Geometry check sheet. Reference: the model listing, model coordinates, mm. Face numbers are marked on the shaded views. A direction names the side the tool comes from. Round coordinates to 2 decimals unless told otherwise and drop trailing zeros. Write each loop counter-clockwise with the first axis right and the second up, starting at its lowest first coordinate (ties: lowest second). Pieces come first, ordered by that corner, then holes. Notation, with made-up numbers: (29, 38.25) -> (72, 38.25) arc R25 ccw to (72, 76.25) -> close; hole circle Ø4 at (49, 4). An arc over 180 degrees is marked (long way). Return JSON: item names as keys, results as strings. Group by question number.
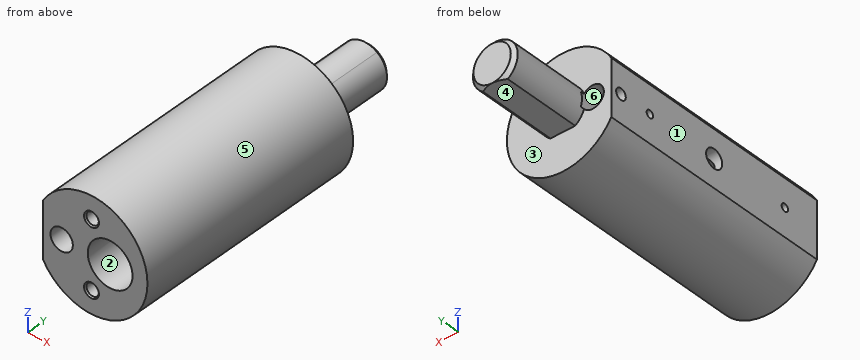
from build123d import *

# Parameters (mm, degrees)
BOSS_EXTRUDE1_DEPTH         = 22
BOSS_EXTRUDE2_DEPTH         = 64
SKETCH3_R                   = 3
CUT_EXTRUDE1_DEPTH          = 65
SKETCH4_R                   = 6
CUT_EXTRUDE2_DEPTH          = 52
M4_TAPPED_HOLE2_D           = 3.3
M4_TAPPED_HOLE2_DEPTH       = 16.8
M4_TAPPED_HOLE2_CSINK_D     = 4
M4_TAPPED_HOLE2_CSINK_ANGLE = 90
M4_TAPPED_HOLE2_TIP         = 0.991420021
SKETCH20_R                  = 2.5
SKETCH20_R_2                = 1.5
CUT_EXTRUDE3_DEPTH          = 5
SKETCH21_R                  = 1
CUT_EXTRUDE4_DEPTH          = 15
BOSS_EXTRUDE4_START         = -22
BOSS_EXTRUDE4_DEPTH         = 22
CUT_EXTRUDE5_DEPTH          = 22
CHAMFER1_SIZE               = 1


with BuildPart() as part:
    # Sketch1 → Boss-Extrude1 (new body)
    with BuildSketch(Plane(origin=(0, 0, 0), x_dir=(1, 0, 0), z_dir=(0, 1, 0))):
        with BuildLine():
            Line((-3.31662479, -5), (3.31662479, -5))
            ThreePointArc((3.31662479, -5), (0, 6), (-3.31662479, -5))
        make_face()
    extrude(amount=BOSS_EXTRUDE1_DEPTH)

    # Sketch2 → Boss-Extrude2 (add)
    with BuildSketch(Plane.XZ):
        with BuildLine():
            Line((-13, 7.483314774), (-13, -7.483314774))
            ThreePointArc((-13, -7.483314774), (15, 0), (-13, 7.483314774))
        make_face()
    extrude(amount=BOSS_EXTRUDE2_DEPTH)

    # Sketch3 → Cut-Extrude1 (cut)
    with BuildSketch(Plane.XZ.offset(64)):
        with Locations(Location((-8, 0, 0), (0, 0, 270))):
            Circle(SKETCH3_R)
    extrude(amount=-CUT_EXTRUDE1_DEPTH, mode=Mode.SUBTRACT)

    # Sketch4 → Cut-Extrude2 (cut)
    with BuildSketch(Plane(origin=(0, -64, 0), x_dir=(-1, 0, 0), z_dir=(0, -1, 0))):
        with Locations(Location((-5, 0, 0), (0, 0, 90))):
            Circle(SKETCH4_R)
    extrude(amount=-CUT_EXTRUDE2_DEPTH, mode=Mode.SUBTRACT)

    # M4 Tapped Hole2
    with Locations(Plane(origin=(0, -64, 0), x_dir=(-1, 0, 0), z_dir=(0, -1, 0))):
        with Locations((0, -9), (0, 9)):
            CounterSinkHole(M4_TAPPED_HOLE2_D / 2, M4_TAPPED_HOLE2_CSINK_D / 2, depth=M4_TAPPED_HOLE2_DEPTH, counter_sink_angle=M4_TAPPED_HOLE2_CSINK_ANGLE)
            with Locations((0, 0, -(M4_TAPPED_HOLE2_DEPTH + M4_TAPPED_HOLE2_TIP / 2))):  # 118° drill point
                Cone(0, M4_TAPPED_HOLE2_D / 2, M4_TAPPED_HOLE2_TIP, mode=Mode.SUBTRACT)

    # Sketch20 → Cut-Extrude3 (cut)
    with BuildSketch(Plane.ZY.offset(13)):
        with Locations((0, -32)):
            Circle(SKETCH20_R)
        with Locations((0, -3)):
            Circle(SKETCH20_R_2)
    extrude(amount=-CUT_EXTRUDE3_DEPTH, mode=Mode.SUBTRACT)

    # Sketch21 → Cut-Extrude4 (cut)
    with BuildSketch(Plane.ZY.offset(13)):
        with Locations((0, -12)):
            Circle(SKETCH21_R)
        with Locations((0, -54)):
            Circle(SKETCH21_R)
    extrude(amount=-CUT_EXTRUDE4_DEPTH, mode=Mode.SUBTRACT)

    # Sketch22 → Boss-Extrude4 (add)
    with BuildSketch(Plane(origin=(0, 22, 0), x_dir=(1, 0, 0), z_dir=(0, 1, 0)).offset(BOSS_EXTRUDE4_START)):
        with BuildLine():
            Line((3.31662479, -5), (-3.31662479, -5))
            ThreePointArc((-3.31662479, -5), (0, -6), (3.31662479, -5))
        make_face()
    extrude(amount=BOSS_EXTRUDE4_DEPTH)

    # Sketch23 → Cut-Extrude5 (cut)
    with BuildSketch(Plane(origin=(0, 22, 0), x_dir=(1, 0, 0), z_dir=(0, 1, 0))):
        Polygon((-67.556784956, 5), (-3.31662479, 5), (3.31662479, 5), (67.556784956, 5), (67.556784956, 133.480320332), (-67.556784956, 133.480320332), align=None)
    extrude(amount=-CUT_EXTRUDE5_DEPTH, mode=Mode.SUBTRACT)

    # Chamfer1
    chamfer1_edges = [part.edges().sort_by_distance(p)[0] for p in [
        (0, 22, 6),
    ]]
    chamfer(chamfer1_edges, length=CHAMFER1_SIZE - 0.0001)  # a hair under: the kernel refuses the full size


solid = part.part
1) Sectioned sample at B-B on x = -8. Enter the section's corners in (y, z).
2) Material ranges on probe 1 along X at (y, z) = (-48, 0); probe 2 along Y at (x, z) = (-11.8, 0); probe 3 along Z at (x, y) = (0, -56.5), recorded low to high. Write a range as [from, to].
3) Mould release check, pull along Z, two halves, no side actions. Record for the marked faces 3, 4, 5 and 6: +Z half, -Z half, draft (parallel to the pull), parting line (faces both ways), or undercut.
4) Sectioned sample at A-A on y = -54. Enter the section's corners in (x, z), and give its area (3 significant figures).
5) Sectioned sample at C-C on z = 0. State how many separate pieces and enclosed holes the cut face has, and give its area (3 significant figures).
6) Tool access check on the marked faces 1 and 2. Record the directions out of +Z, -Z, +X, -X, +Y, -Y that give a thin tool (end or side, any length) a straight path to the whole face; none if there is none.
7) Sectioned sample at D-D on y = -3. Enter the section's corners in (x, z), and give its area (3 significant figures).
8) Go/stop test with flat-tipped pins: P1, Ø10, axis at x = 5.5, y = -17, coming from the -Z side; P2, Ø2, axis at y = -15, z = 11.5, coming from the +X side; P3, Ø1, axis at x = 9, z = -9.5, coming from the +Y side. Record where each tip stops, or that it passes through.
Evaluation:
{
 "1": {"outline": "(-64, -12.69) -> (0, -12.69) -> (0, -3) -> (-64, -3) -> close; (-64, 3) -> (0, 3) -> (0, 12.69) -> (-64, 12.69) -> close"},
 "2": {"probe 1": "x = [-13, -11], [-5, -1], [11, 15]", "probe 2": "y = [-64, -55], [-53, -34.5], [-29.5, -13], [-11, -4.5], [-1.5, 0]", "probe 3": "z = [-15, -10.65], [-7.35, -3.32], [3.32, 7.35], [10.65, 15]"},
 "3": {"face 3": "draft", "face 4": "-Z half", "face 5": "parting line", "face 6": "undercut"},
 "4": {"outline": "(-13, -7.48) arc R15 ccw (long way) to (-13, 7.48) -> (-13, 1) -> (-10.83, 1) arc R3 cw to (-5.17, 1) -> (-0.92, 1) arc R6 cw (long way) to (-0.92, -1) -> (-5.17, -1) arc R3 cw to (-10.83, -1) -> (-13, -1) -> close; hole circle Ø3.3 at (0, -9); hole circle Ø3.3 at (0, 9)", "area": "516 mm2"},
 "5": {"separate pieces": "8", "enclosed holes": "0", "area": "1,000 mm2"},
 "6": {"face 1": "+Z, -Z, -X, +Y, -Y", "face 2": "-Y"},
 "7": {"outline": "(-13, -7.48) arc R15 ccw (long way) to (-13, 7.48) -> (-13, 1.5) -> (-10.6, 1.5) arc R3 cw (long way) to (-10.6, -1.5) -> (-13, -1.5) -> close", "area": "652 mm2"},
 "8": {"P1": "stops at z = -14.99", "P2": "stops at x = 10.71", "P3": "stops at y = 0"}
}
